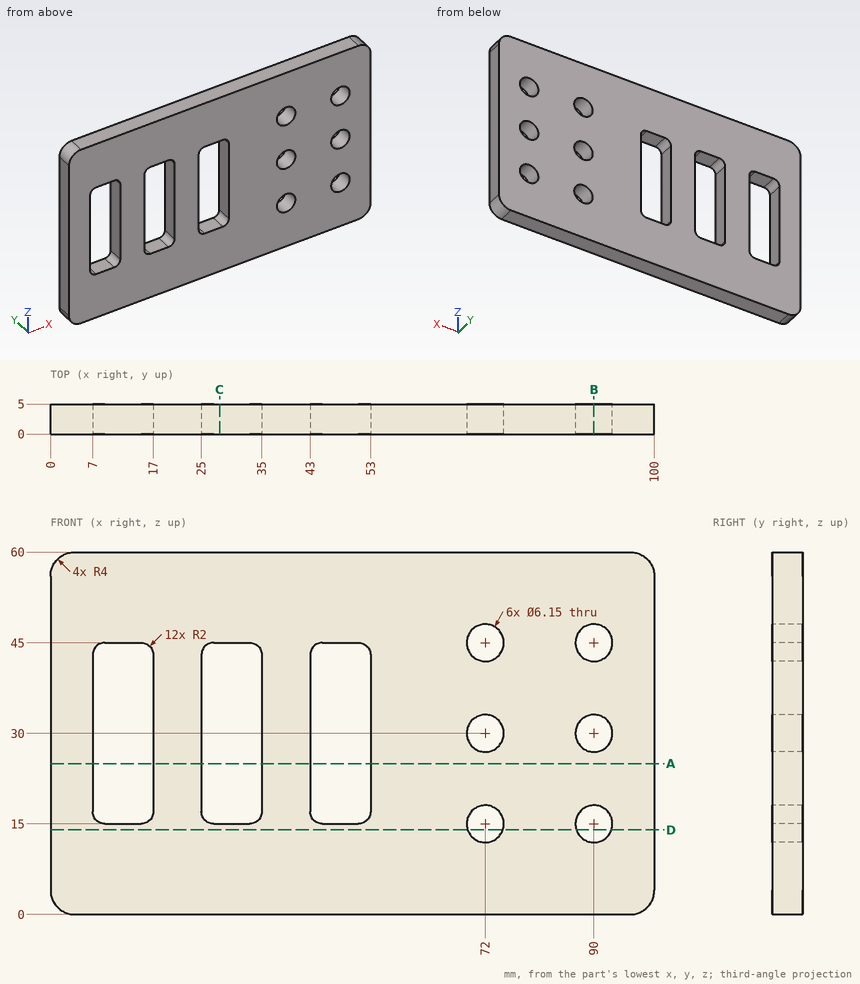
Drawing for the job (mm, zero at the part's lowest x, y, z). Coordinates: 2 decimals unless noted, no trailing zeros. Write each loop counter-clockwise with the first axis right and the second up, starting at its lowest first coordinate (ties: lowest second). Pieces come first, ordered by that corner, then holes. Notation, with made-up numbers: (58, 46.25) -> (92, 46.25) arc R29 cw to (92, 82.25) -> close; hole circle Ø7 at (-0.5, -18.5). An arc over 180 degrees is marked (long way). One line per item, written item: value. Start each with the question number.
1) Slice it at D-D on z = 14. Write the cut outline in (x, y), then the cut area to 3 significant figures.
2) Probe probe 1 along Z at (x, y) = (72, 2.95) (3 decimals); probe 2 along X at (y, z) = (1.4, 41.5); probe 3 along Z at (x, y) = (45, 0.9). List the from-to ranges inside material, lowest first.
3) Slice it at B-B on x = 90. Write the cut outline in (y, z) (3 decimals), then the cut area to 3 significant figures.
4) Flat gauge pin, fed straight in: pin 1 Ø5 at (x, z) = (72, 30) entering from +Y. Where does the tip first touch, or does it go through?
5) Slice it at A-A on z = 25. Write the cut outline in (x, y), then the cut area to 3 significant figures.
6) Slice it at C-C on x = 28. Write the cut outline in (y, z), then the cut area to 3 significant figures.
Answers follow:
1. outline: (0, 0) -> (69.09, 0) -> (69.09, 5) -> (0, 5) -> close; (74.91, 0) -> (87.09, 0) -> (87.09, 5) -> (74.91, 5) -> close; (92.91, 0) -> (100, 0) -> (100, 5) -> (92.91, 5) -> close
1. area: 442 mm2
2. probe 1: 0 to 11.925, 18.075 to 26.925, 33.075 to 41.925, 48.075 to 60
2. probe 2: 0 to 7, 17 to 25, 35 to 43, 53 to 100
2. probe 3: 0 to 15, 45 to 60
3. outline: (0, 0) -> (5, 0) -> (5, 11.925) -> (0, 11.925) -> close; (0, 18.075) -> (5, 18.075) -> (5, 26.925) -> (0, 26.925) -> close; (0, 33.075) -> (5, 33.075) -> (5, 41.925) -> (0, 41.925) -> close; (0, 48.075) -> (5, 48.075) -> (5, 60) -> (0, 60) -> close
3. area: 208 mm2
4. pin 1: through
5. outline: (0, 0) -> (7, 0) -> (7, 5) -> (0, 5) -> close; (17, 0) -> (25, 0) -> (25, 5) -> (17, 5) -> close; (35, 0) -> (43, 0) -> (43, 5) -> (35, 5) -> close; (53, 0) -> (100, 0) -> (100, 5) -> (53, 5) -> close
5. area: 350 mm2
6. outline: (0, 0) -> (5, 0) -> (5, 15) -> (0, 15) -> close; (0, 45) -> (5, 45) -> (5, 60) -> (0, 60) -> close
6. area: 150 mm2
